from build123d import *

# Parameters (mm, degrees)
F0_R     = 762
F1_DEPTH = 50.8
F2_W     = 50.8
F2_H     = 25.4
F3_DEPTH = 685.8


with BuildPart() as f1:
    # F0 (on Top) → F1 (new body)
    with BuildSketch(Plane.XY):
        Circle(F0_R)
    extrude(amount=F1_DEPTH)

    # F2 (on face) → F3 (join)
    with BuildSketch(Plane(origin=(0, 0, 0), x_dir=(1, 0, 0), z_dir=(0, 0, -1))):
        with Locations((-444.5, 508)):
            Rectangle(F2_W, F2_H)
        with Locations((444.5, 508)):
            Rectangle(F2_W, F2_H)
        with Locations((-444.5, -508)):
            Rectangle(F2_W, F2_H)
        with Locations((444.5, -508)):
            Rectangle(F2_W, F2_H)
    extrude(amount=F3_DEPTH)


solid = f1.part
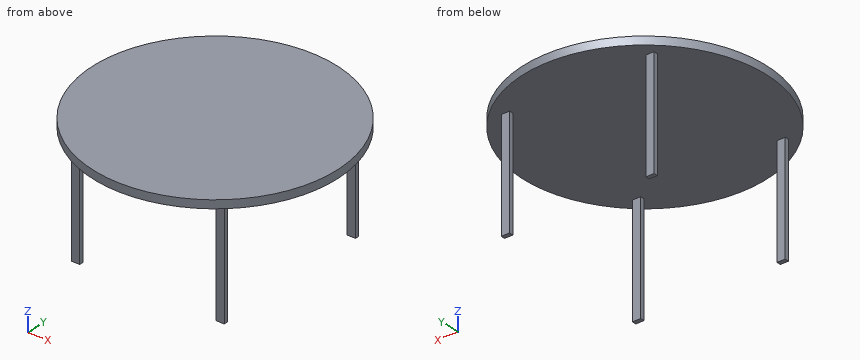
Verification items for the finished model (mm, model axes). Give positions to 0.01 mm unless a question says otherwise; leave off trailing zeros. Write each loop counter-clockwise with the first axis right and the second up, starting at its lowest first coordinate (ties: lowest second). Pieces come first, ordered by that corner, then holes.
(1) Material ranges on line 1 (Y direction, x = -452.5, z = -233.5); line 2 (X direction, y = -519, z = -492); line 3 (Z direction, x = 29, y = 222), recorded low to high.
(2) Gauge pin test, flat ends, axial feed: pin 1 (20.5 mm diameter, centred on y = -506, z = -428.5, fed in from +X); pin 2 (15 mm diameter, centred on x = -451, z = -468.5, fed in from -Y); pin 3 (12.5 mm diameter, centred on y = 504.5, z = -433.5, fed in from -X). Record the tip position at first contact, or that the pin passes through.
(3) Cross-section at A-A (z = -432.5). Enter the section's corners in (x, y).
(4) Cross-section at B-B (x = 0). Enter the section's corners in (y, z).
Worked out:
1. line 1: y = -520.7 to -495.3, 495.3 to 520.7
1. line 2: x = -469.9 to -419.1, 419.1 to 469.9
1. line 3: z = 0 to 50.8
2. pin 1: stops at x = 469.9
2. pin 2: stops at y = -520.7
2. pin 3: stops at x = -469.9
3. outline: (-469.9, -520.7) - (-419.1, -520.7) - (-419.1, -495.3) - (-469.9, -495.3) - close; (-469.9, 495.3) - (-419.1, 495.3) - (-419.1, 520.7) - (-469.9, 520.7) - close; (419.1, -520.7) - (469.9, -520.7) - (469.9, -495.3) - (419.1, -495.3) - close; (419.1, 495.3) - (469.9, 495.3) - (469.9, 520.7) - (419.1, 520.7) - close
4. outline: (-762, 0) - (762, 0) - (762, 50.8) - (-762, 50.8) - close
